from build123d import *

# Parameters (mm, degrees)
F0_W     = 127
F0_H     = 101.6
F1_DEPTH = 76.2
F3_DEPTH = 101.6
F4_W     = 7.62
F4_H     = 5.08
F5_DEPTH = 76.2


with BuildPart() as f1:
    # F0 (on Top) → F1 (new body)
    with BuildSketch(Plane.XY):
        with Locations((22.224299, -15.116411)):
            Rectangle(F0_W, F0_H)
    extrude(amount=F1_DEPTH)

    # F2 (on face) → F3 (join)
    with BuildSketch(Plane.XZ.offset(65.916411)):
        Polygon((152.926383, 0), (85.724299, 76.2), (85.724299, 0), align=None)
    extrude(amount=-F3_DEPTH)

    # F4 (on face) → F5 (join)
    with BuildSketch(Plane(origin=(0, 0, 0), x_dir=(1, 0, 0), z_dir=(0, 0, -1))):
        with Locations((-45.085701, -15.363589)):
            Rectangle(F4_W, F4_H)
        with BuildLine():
            ThreePointArc((-48.895701, 48.136411), (-58.37511, 45.596411), (-48.895701, 43.056411))
            Line((-48.895701, 43.056411), (-48.895701, 48.136411))
        make_face()
        with Locations((-45.085701, 45.596411)):
            Rectangle(F4_W, F4_H)
        with BuildLine():
            ThreePointArc((-48.895701, 17.656411), (-58.37511, 15.116411), (-48.895701, 12.576411))
            Line((-48.895701, 12.576411), (-48.895701, 17.656411))
        make_face()
        with Locations((-45.085701, 15.116411)):
            Rectangle(F4_W, F4_H)
        with BuildLine():
            ThreePointArc((-48.895701, -12.823589), (-58.37511, -15.363589), (-48.895701, -17.903589))
            Line((-48.895701, -17.903589), (-48.895701, -12.823589))
        make_face()
    extrude(amount=-F5_DEPTH)


solid = f1.part
Geometry: final body of the model. Coordinates: model frame, mm. A direction names the side the tool comes from. Round coordinates to 2 decimals unless told otherwise and drop trailing zeros. Order: outer loops, then holes, each group sorted by start corner. A loop starts at its lowest first (then second) coordinate and runs counter-clockwise, first axis right, second up. Notation, with made-up numbers: (75, 65.25) - (85, 65.25) arc R22 ccw to (85, 79.25) - close; hole circle Ø9 at (39, -1.75). An arc over 180 degrees is marked (long way). Write each question's results on one line, items separated by ' | '.
Item 1: Section C-C, the plane x = 126. Return the cut outline in (y, z), and give its area (3 significant figures).
Completed:
outline: (-65.92, 0) - (35.68, 0) - (35.68, 30.53) - (-65.92, 30.53) - close | area: 3,100 mm^2
Item 2: Section B-B, the plane y = -32. Return the cut outline in (x, z), and give its area (3 significant figures).
Completed:
outline: (-41.28, 0) - (152.93, 0) - (85.72, 76.2) - (-41.28, 76.2) - close | area: 12,200 mm^2
Item 3: Material intervals for line 1 along X through (y, z) = (-49, 5.5); line 2 along X through (y, z) = (-50, 24); line 3 along Z through (x, y) = (125.5, 24), sorted ascending. Write a range as [from, to].
Completed:
line 1: [-57.07, -49.52], [-41.28, 148.08] | line 2: [-55.83, -50.76], [-41.28, 131.76] | line 3: [0, 31.1]
Item 4: Section D-D, the plane z = 24. Return the cut outline in (x, y).
Completed:
outline: (-48.9, -48.14) - (-41.28, -48.14) - (-41.28, -65.92) - (131.76, -65.92) - (131.76, 35.68) - (-41.28, 35.68) - (-41.28, 17.9) - (-48.9, 17.9) arc R5.08 ccw (long way) to (-48.9, 12.82) - (-41.28, 12.82) - (-41.28, -12.58) - (-48.9, -12.58) arc R5.08 ccw (long way) to (-48.9, -17.66) - (-41.28, -17.66) - (-41.28, -43.06) - (-48.9, -43.06) arc R5.08 ccw (long way) to start
Item 5: Reachability of faces 1 (the flat face through (-45, -48.136, 38)), 2 (the flat face through (-45, -12.576, 38)), 3 (the flat face through (33, 35.684, 39)), 4 (the flat face through (-45, 17.904, 38)) from +Z, -Z, +X, -X, +Y, -Y: full face, straight path, thin tool, end or side. Return the list, or none.
Completed:
face 1: +Z, -Z, -Y | face 2: +Z, -Z | face 3: +Z, -Z, +X, -X, +Y | face 4: +Z, -Z, +Y
Item 6: Section A-A, the plane z = 44.5. Return the cut outline in (x, y), and give its area (3 significant figures).
Completed:
outline: (-48.9, -48.14) - (-41.28, -48.14) - (-41.28, -65.92) - (113.68, -65.92) - (113.68, 35.68) - (-41.28, 35.68) - (-41.28, 17.9) - (-48.9, 17.9) arc R5.08 ccw (long way) to (-48.9, 12.82) - (-41.28, 12.82) - (-41.28, -12.58) - (-48.9, -12.58) arc R5.08 ccw (long way) to (-48.9, -17.66) - (-41.28, -17.66) - (-41.28, -43.06) - (-48.9, -43.06) arc R5.08 ccw (long way) to start | area: 16,100 mm^2
Item 7: Mould query, pull axis X, two halves, no side actions, for faces 5 (the flat face through (119.796, -15.828, 37.567)), 6 (the flat face through (46, -16, 0)), 7 (the cylindrical face through (-58.37, 15.18, 37.57)). Classes: pulls with the +X half, pulls with the -X half, needs draft (parallel to the pull), parting line crosses it, or undercut.
Completed:
face 5: pulls with the +X half | face 6: needs draft | face 7: undercut
Item 8: First-contact query: pin 1 Ø4 at (x, z) = (-47, 55) entering from +Y; pin 2 Ø6 at (y, z) = (-8.5, 14.5) entering from -X; pin 3 Ø5.5 at (y, z) = (-54, 23) entering from -X. Flat tips, straight axial feed; report the tip coordinate or a pass-through.
Completed:
pin 1: y = 18.08 | pin 2: x = -56.86 | pin 3: x = -41.28
